Can you work these out from the model? Positions are in its coordinate system, mm. Face numbers are marked on the shaded views. A direction names the side the tool comes from. Round coordinates to 2 decimals unless told otherwise and drop trailing zeros. Order: outer loops, then holes, each group sorted by start corner. A loop starts at its lowest first (then second) coordinate and runs counter-clockwise, first axis right, second up. Notation, with made-up numbers: (-3.5, -31.5) -> (16.5, -31.5) arc R18 cw to (16.5, -20.5) -> close; hole circle Ø8 at (-27, 80). An arc over 180 degrees is marked (long way). Use a Markdown table: item, result. Add a question column.
Q1. If we section it at B-B on x = 11.5: List the corners of the cut face in (y, z) for me.
Q2. For the marked faces 5 and 6, which set-ups out of +Z, -Z, +X, -X, +Y, -Y let a thin tool reach every point of the face, with its end or its side?
Q3. I'm going to push flat-ended pins straight in: pin 1 Ø0.6 at (x, z) = (-25, -18.5) entering from +Y; pin 2 Ø2 at (x, y) = (-27, 9.5) entering from +Z; pin 3 Ø1 at (y, z) = (10.5, -32) entering from -X. Where does each tip first touch, or does it pass through?
Q4. If we section it at A-A on z = -19.1: List the corners of the cut face in (x, y) for me.
Q5. If we section it at C-C on z = 10: List the corners of the cut face in (x, y) for me, plus the area to 3 significant figures.
Q6. We'd pull the mould along Z, two halves only. Please class the marked faces 1, 2, 3 and 4: +Z half, -Z half, draft (parallel to the pull), parting line (faces both ways), or undercut.
Q7. I need wall thicknesses on line 1 along X through (y, z) = (10.25, -19.1); line 2 along Z through (x, y) = (-13.5, 12.75); line 3 along Z through (x, y) = (1.5, 11.25). Which ranges of each line are inside material? Lowest first, please. Write a range as [from, to].
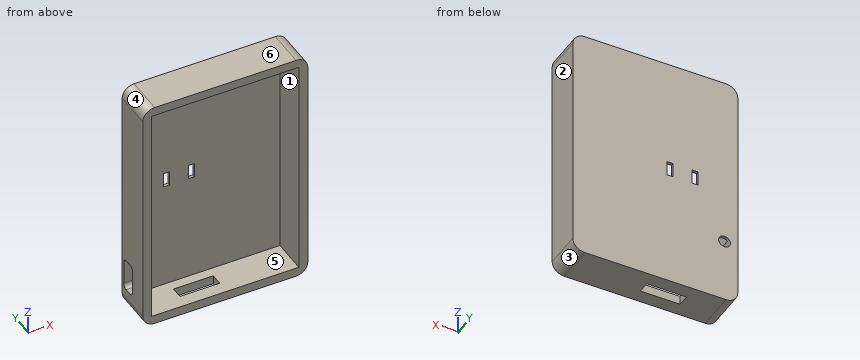
Autodesk Inventor part; units mm, degrees
ref_plane "YZ Plane" through (0, 0, 0) normal (1, 0, 0) x (0, 1, 0)
ref_plane "XZ Plane" through (0, 0, 0) normal (0, 1, 0) x (-1, 0, 0)
ref_plane "XY Plane" through (0, 0, 0) normal (0, 0, 1) x (1, 0, 0)
sketch "Boceto1" plane through (0, 0, 0) normal (0, 1, 0) x (-1, 0, 0)
  line L0 (-25, 38) -> (25, 38)
  line L1 (25, 38) -> (25, -38)
  line L2 (25, -38) -> (-25, -38)
  line L3 (-25, -38) -> (-25, 38)
  line L4 (-25, 38) -> (25, -38) construction
  line L5 (25, 38) -> (-25, -38) construction
  line L6 (28, -37) -> (28, 37)
  line L7 (24, 41) -> (-24, 41)
  line L8 (-28, 37) -> (-28, -37)
  line L9 (-24, -41) -> (24, -41)
  arc A0 (28, 37) -> (24, 41) centre (24, 37) ccw
  arc A1 (24, -41) -> (28, -37) centre (24, -37) ccw
  arc A2 (-28, -37) -> (-24, -41) centre (-24, -37) ccw
  arc A3 (-24, 41) -> (-28, 37) centre (-24, 37) ccw
  point P0 (0, 0)
  dimension "d0" = 50
  dimension "d1" = 76
  dimension "d2" = 3
  dimension "d3" = 4
extrude "Extrusión1" add sketch "Boceto1" along normal blind 12
sketch "Boceto2" plane through (0, 12, 0) normal (0, 1, 0) x (1, 0, 0)
  arc A0 (-28, -37) -> (-24, -41) centre (-24, -37) ccw
  line L0 (-24, -41) -> (24, -41)
  arc A1 (24, -41) -> (28, -37) centre (24, -37) ccw
  line L1 (28, -37) -> (28, 37)
  arc A2 (28, 37) -> (24, 41) centre (24, 37) ccw
  line L2 (24, 41) -> (-24, 41)
  arc A3 (-24, 41) -> (-28, 37) centre (-24, 37) ccw
  line L3 (-28, 37) -> (-28, -37)
  line L4 (25, -38) -> (-25, -38)
  line L5 (-25, -38) -> (-25, 38)
  line L6 (-25, 38) -> (25, 38)
  line L7 (25, 38) -> (25, -38)
  point P0 (0, 0)
extrude "Extrusión2" add sketch "Boceto2" along normal blind 1 contours L3 A3 L2 A2 L1 A1 L0 A0 | L4 L5 L6 L7
sketch "Boceto3" plane through (25, 0, -38) normal (-1, 0, 0) x (0, 0, 1)
  line L0 (0, 0) -> (76, 0)
  line L1 (76, 0) -> (76, 12)
  line L2 (0, 12) -> (76, 12)
  line L3 (0, 0) -> (0, 12)
  line L4 (5.5, 12) -> (13.5, 12)
  line L5 (15, 10.5) -> (15, 8)
  line L6 (13.5, 6.5) -> (5.5, 6.5)
  line L7 (4, 8) -> (4, 10.5)
  arc A0 (13.5, 6.5) -> (15, 8) centre (13.5, 8) ccw
  arc A1 (4, 8) -> (5.5, 6.5) centre (5.5, 8) ccw
  arc A2 (15, 10.5) -> (13.5, 12) centre (13.5, 10.5) ccw
  arc A3 (5.5, 12) -> (4, 10.5) centre (5.5, 10.5) ccw
  point P0 (38, 0)
  point P1 (15, 12)
  point P2 (15, 6.5)
  point P3 (4, 6.5)
  point P4 (4, 12)
  point P5 (13.5, 12)
  point P6 (5.5, 12)
  dimension "d8" = 15
  dimension "d9" = 5.5
  dimension "d10" = 11
  dimension "d11" = 90
  dimension "d12" = 5.5
  dimension "d13" = 90
  dimension "d14" = 1.5
  dimension "d15" = 1.5
extrude "Extrusión3" cut sketch "Boceto3" along normal through all contours L2 A2 L5 A0 L6 A1 L7 A3
sketch "Boceto4" plane through (-25, 0, -38) normal (0, 0, 1) x (1, 0, 0)
  line L0 (0, 0) -> (50, 0)
  line L1 (50, 0) -> (50, 12)
  line L2 (0, 12) -> (50, 12)
  line L3 (0, 0) -> (0, 12)
  line L4 (0, 12) -> (25.5, 12)
  line L5 (25.5, 12) -> (25.5, 4.5)
  line L6 (25.5, 4.5) -> (12, 4.5)
  line L7 (25.5, 12) -> (25.5, 8.5)
  line L8 (25.5, 8.5) -> (12, 8.5)
  line L9 (12, 8.5) -> (12, 4.5)
  point P0 (25, 0)
  dimension "d18" = 25.5
  dimension "d19" = 7.5
  dimension "d20" = 13.5
  dimension "d21" = 3.5
extrude "Extrusión4" cut sketch "Boceto4" against normal blind 10 contours L5 L6 L9 L8
sketch "Boceto5" plane through (0, 12, 0) normal (0, -1, 0) x (1, 0, 0)
  line L0 (-25, -32.5) -> (-25, -38)
  line L1 (-25, -38) -> (25, -38)
  line L2 (25, -38) -> (25, 38)
  line L3 (25, 38) -> (-25, 38)
  line L4 (-25, 38) -> (-25, -24.5)
  line L5 (-25, -24.5) -> (-28, -24.5)
  line L6 (-28, -32.5) -> (-28, -24.5)
  line L7 (-25, -32.5) -> (-28, -32.5)
  line L8 (-25, -23) -> (-25, -24.5)
  line L9 (-25, 38) -> (-25, -24.5)
  line L10 (-25, 38) -> (-25, -38)
  line L11 (-25, -32.5) -> (-25, -38)
  line L12 (-25, -32.5) -> (-25, -34)
  line L13 (-25, -34) -> (-25, -32.5)
  line L14 (-25, -32.5) -> (-25, -24.5)
  line L15 (-25, -24.5) -> (-25, -23)
  line L16 (-25, -23) -> (-25, -19.1)
  line L17 (-25, -23) -> (-21.1, -23) construction
  line L18 (-25, -19.1) -> (-23.5, -19.1)
  circle A0 centre (-23.5, -19.1) radius 2
  point P0 (0, 0)
  dimension "d24" = 3.9
  dimension "d25" = 90
  dimension "d26" = 1.5
  dimension "d27" = 4
extrude "Extrusión5" cut sketch "Boceto5" along normal mid plane 14 contours A0 L4 | L4 A0
sketch "Boceto6" plane through (0, 12, 0) normal (0, -1, 0) x (1, 0, 0)
  arc A0 (-25, -20.4229) -> (-25, -17.7771) centre (-23.5, -19.1) ccw
  line L0 (-25, -20.4229) -> (-25, -24.5)
  line L1 (-25, -24.5) -> (-28, -24.5)
  line L2 (-28, -32.5) -> (-28, -24.5)
  line L3 (-25, -32.5) -> (-28, -32.5)
  line L4 (-25, -32.5) -> (-25, -38)
  line L5 (-25, -38) -> (25, -38)
  line L6 (25, -38) -> (25, 38)
  line L7 (25, 38) -> (-25, 38)
  line L8 (-25, 38) -> (-25, -17.7771)
  line L9 (-6, 4) -> (-4, 4)
  line L10 (-4, 4) -> (-4, -1)
  line L11 (-4, -1) -> (-6, -1)
  line L12 (-6, -1) -> (-6, 4)
  line L13 (-6, 4) -> (-4, -1) construction
  line L14 (-4, 4) -> (-6, -1) construction
  line L15 (-14.5, 4) -> (-12.5, 4)
  line L16 (-12.5, 4) -> (-12.5, -1)
  line L17 (-12.5, -1) -> (-14.5, -1)
  line L18 (-14.5, -1) -> (-14.5, 4)
  line L19 (-14.5, 4) -> (-12.5, -1) construction
  line L20 (-12.5, 4) -> (-14.5, -1) construction
  point P0 (0, 0)
  point P1 (-13.5, 1.5)
  point P2 (-5, 1.5)
  dimension "d30" = 11.5
  dimension "d31" = 39.5
  dimension "d32" = 8.5
  dimension "d33" = 2
  dimension "d34" = 5
  dimension "d35" = 2
  dimension "d36" = 5
extrude "Extrusión6" cut sketch "Boceto6" against normal blind 14 contours L9 L10 L11 L12 | L15 L16 L17 L18
properties part number "Pieza1_3DPrint"
Answer below:
| question | item | result |
|---|---|---|
| 1 | outline | (0, -41) -> (13, -41) -> (13, 41) -> (0, 41) -> (0, 38) -> (12, 38) -> (12, -38) -> (0, -38) -> close |
| 2 | face 5 | -Y |
| 2 | face 6 | +Z, +X, -X, +Y, -Y |
| 3 | pin 1 | y = 5 |
| 3 | pin 2 | z = 40.46 |
| 3 | pin 3 | x = 25 |
| 4 | outline | (-28, 0) -> (-25, 0) -> (-25, 5) -> (-25.5, 5) -> (-25.5, 13) -> (-28, 13) -> close; (-21.5, 12) -> (25, 12) -> (25, 0) -> (28, 0) -> (28, 13) -> (-21.5, 13) -> close |
| 5 | outline | (-28, 0) -> (-25, 0) -> (-25, 12) -> (25, 12) -> (25, 0) -> (28, 0) -> (28, 13) -> (-28, 13) -> close |
| 5 | area | 128 mm² |
| 6 | face 1 | undercut |
| 6 | face 2 | draft |
| 6 | face 3 | -Z half |
| 6 | face 4 | +Z half |
| 7 | line 1 | [-28, -25.5], [25, 28] |
| 7 | line 2 | [-41, -1], [4, 41] |
| 7 | line 3 | [-41, -38], [38, 41] |
